Verification items for the finished model (mm, model axes). A direction names the side the tool comes from. Round coordinates to 2 decimals unless told otherwise and drop trailing zeros. Write each loop counter-clockwise with the first axis right and the second up, starting at its lowest first coordinate (ties: lowest second). Pieces come first, ordered by that corner, then holes. Notation, with made-up numbers: M 48,58.25 L 104,58.25 A6 ccw 104,68.25 Z; hole C -28.75,87 d5. An arc over 180 degrees is marked long. One line per question, with ' | ' between items. Start each with the question number.
Q1. Tool access check on faces 4 (the face through (100, 10, 10)), 5 (the face through (32.253, 0.121, 23.944)). Record the directions out of +Z, -Z, +X, -X, +Y, -Y that give a thin tool (end or side, any length) a straight path to the whole face; none if there is none.
Q2. Cross-section at C-C (x = 46). Record the boundary of the cut face in (y, z).
Q3. Release check for a two-part mould opening along X. For faces 1 (the face through (-1, -22, 28)), 2 (the face through (285, 0, 10)), 3 (the face through (130, 0, 10)) record: released by +X, released by -X, zero draft, split by the parting line, or undercut.
Q4. Thickness scan on line 1 along Y through (x, z) = (0, 12.5); line 2 along Z through (x, y) = (214.5, -23); line 3 along X through (y, z) = (5, 15.25). Record the ranges inside material, lowest first. Write a range as from..to.
Q5. Cross-section at B-B (z = 23). Record the boundary of the cut face in (x, y).
Q6. Cross-section at A-A (x = 0). Record the boundary of the cut face in (y, z).
Q7. Cross-section at D-D (z = 5.75). State how many separate pieces and enclosed holes the cut face has, then the cut area to 3 significant figures.
Q8. Gauge pin test, flat ends, axial feed: pin 1 (6 mm diameter, centred on x = 114, z = 9.5, fed in from -Y); pin 2 (10 mm diameter, centred on y = 1.5, z = 12.5, fed in from -X); pin 3 (6 mm diameter, centred on y = 34, z = 11.5, fed in from -X). Record the tip position at first contact, or that the pin passes through.
from build123d import *

# Parameters (mm, degrees)
SKETCH1_R           = 50
SKETCH1_R_2         = 17.5
SKETCH1_R_3         = 2.75
BOSS_EXTRUDE1_DEPTH = 28
SKETCH3_W           = 60
SKETCH3_H           = 20
SKETCH3_H_2         = 16
BOSS_EXTRUDE3_DEPTH = 20


with BuildPart() as part:
    # Sketch1 → Boss-Extrude1 (new body)
    with BuildSketch(Plane.XY):
        Circle(SKETCH1_R)
        Circle(SKETCH1_R_2, mode=Mode.SUBTRACT)
        with Locations((35, 0)):
            Circle(SKETCH1_R_3, mode=Mode.SUBTRACT)
        with Locations((17.5, 30.310889132)):
            Circle(SKETCH1_R_3, mode=Mode.SUBTRACT)
        with Locations((-17.5, 30.310889132)):
            Circle(SKETCH1_R_3, mode=Mode.SUBTRACT)
        with Locations((-35, 0)):
            Circle(SKETCH1_R_3, mode=Mode.SUBTRACT)
        with Locations((-17.5, -30.310889132)):
            Circle(SKETCH1_R_3, mode=Mode.SUBTRACT)
        with Locations((17.5, -30.310889132)):
            Circle(SKETCH1_R_3, mode=Mode.SUBTRACT)
    extrude(amount=BOSS_EXTRUDE1_DEPTH)

    # Sketch3 → Boss-Extrude3 (add)
    with BuildSketch(Plane.XY):
        Polygon((15, -28), (15, 28), (285, 22), (285, -22), align=None)
        with Locations((100, 0)):
            Rectangle(SKETCH3_W, SKETCH3_H, mode=Mode.SUBTRACT)
        with Locations((200, 0)):
            Rectangle(SKETCH3_W, SKETCH3_H_2, mode=Mode.SUBTRACT)
    extrude(amount=BOSS_EXTRUDE3_DEPTH)


solid = part.part
Determined:
1) face 4: +Z, -Z | face 5: +Z
2) outline: M -27.31,0 L 27.31,0 L 27.31,20 L 19.6,20 L 19.6,28 L -19.6,28 L -19.6,20 L -27.31,20 Z
3) face 1: zero draft | face 2: released by +X | face 3: undercut
4) line 1: y = -50..-17.5, 17.5..50 | line 2: z = 0..20 | line 3: x = -49.75..-16.77, 15..70, 130..170, 230..285
5) outline: C 0,0 d100; hole C -35,0 d5.5; hole C -17.5,-30.31 d5.5; hole C -17.5,30.31 d5.5; hole C 0,0 d35; hole C 17.5,-30.31 d5.5; hole C 17.5,30.31 d5.5; hole C 35,0 d5.5
6) outline: M -50,0 L -17.5,0 L -17.5,28 L -50,28 Z; M 17.5,0 L 50,0 L 50,28 L 17.5,28 Z
7) separate pieces: 1 | enclosed holes: 8 | area: 16,400 mm²
8) pin 1: stops at y = -25.87 | pin 2: stops at x = -50 | pin 3: stops at x = -39.23
